The model under review builds one solid part; all positions refer to its coordinate system, in mm. Face numbers are marked on the shaded views. Round coordinates to 2 decimals unless told otherwise and drop trailing zeros. Write each loop counter-clockwise with the first axis right and the second up, starting at its lowest first coordinate (ties: lowest second). Pieces come first, ordered by that corner, then holes. Notation, with made-up numbers: (42, 62.5) - (60, 62.5) arc R17 cw to (60, 92.5) - close; hole circle Ø11 at (-38, -18). An arc over 180 degrees is marked (long way). Return JSON: item names as keys, results as strings.
from build123d import *

# Parameters (mm, degrees)
SKETCH1_R          = 4.5
INSERT_SHAPE_DEPTH = 9
SKETCH3_R          = 2.5
CENTER_HOLE_DEPTH  = 4.3
TAPPED_HOLE_REACH  = 9.911
SKETCH4_R          = 1.75


with BuildPart() as part:
    # Sketch1 → insert shape (new body)
    with BuildSketch(Plane.XY):
        Circle(SKETCH1_R)
    extrude(amount=INSERT_SHAPE_DEPTH)

    # Sketch3 → center hole (cut)
    with BuildSketch(Plane.XY.offset(9)):
        Circle(SKETCH3_R)
    extrude(amount=-CENTER_HOLE_DEPTH, mode=Mode.SUBTRACT)

    # Sketch4 → tapped hole (cut, up to next)
    with BuildSketch(Plane.XY.offset(4.7), mode=Mode.PRIVATE) as tapped_hole_sk1:
        Circle(SKETCH4_R)
    tapped_hole_tool1 = extrude(tapped_hole_sk1.sketch, amount=-TAPPED_HOLE_REACH, mode=Mode.PRIVATE) & part.part
    add(tapped_hole_tool1.solids().sort_by_distance((0, 0, 4.7))[0], mode=Mode.SUBTRACT)


solid = part.part
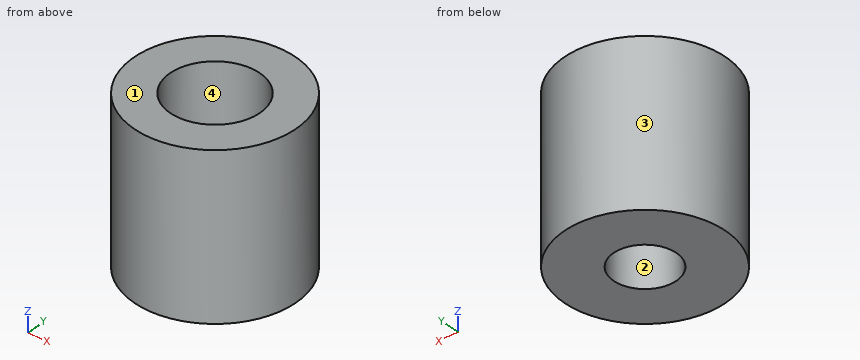
(1) Add section A-A (x = 0). Write out the cut boundary in (y, z).
Filled in:
{"outline": "(-4.5, 0) - (-1.75, 0) - (-1.75, 4.7) - (-2.5, 4.7) - (-2.5, 9) - (-4.5, 9) - close; (1.75, 0) - (4.5, 0) - (4.5, 9) - (2.5, 9) - (2.5, 4.7) - (1.75, 4.7) - close"}
(2) Add section D-D (z = 4.25). Write out the cut boundary in (x, y).
Filled in:
{"outline": "circle Ø9 at (0, 0); hole circle Ø3.5 at (0, 0)"}
(3) Mouldability with a two-part tool opening along Y and no side actions: class the marked faces 1, 2, 3 and 4 as released by +Y, released by -Y, zero draft, split by the parting line, or undercut.
Filled in:
{"face 1": "zero draft", "face 2": "undercut", "face 3": "split by the parting line", "face 4": "undercut"}
(4) Wall thickness on line 1 (Y direction, x = 0, z = 5.6); line 2 (Z direction, x = 0.5, y = -2); line 3 (X direction, y = 0.25, z = 7.75): over which ranges is each line inside the solid? List them lowest first.
Filled in:
{"line 1": "y = -4.5 to -2.5, 2.5 to 4.5", "line 2": "z = 0 to 4.7", "line 3": "x = -4.49 to -2.49, 2.49 to 4.49"}
(5) Add section C-C (z = 7.25). Write out the cut boundary in (x, y), plus the area to 3 significant figures.
Filled in:
{"outline": "circle Ø9 at (0, 0); hole circle Ø5 at (0, 0)", "area": "44.0 mm2"}
(6) Clearance check with flat-ended pins moving along their axes: pin 1 Ø1.5 at (y, z) = (-2.5, 5) entering from -X; pin 2 Ø1 at (y, z) = (-3.5, 5.5) entering from +X; pin 3 Ø3 at (y, z) = (-3.5, 4.5) entering from -X. State where each tip first meets the part, or that it passes through.
Filled in:
{"pin 1": "stops at x = -4.15", "pin 2": "stops at x = 3.35", "pin 3": "stops at x = -4.03"}
